Input: dimensioned drawing with shaded views. Units: mm. Origin: part minimum x, y, z. Coordinates: 2 decimals unless noted, no trailing zeros. Order: outer loops, then holes, each group sorted by start corner. A loop starts at its lowest first (then second) coordinate and runs counter-clockwise, first axis right, second up. Notation, with made-up numbers: (-33.75, 51.25) -> (-11.75, 51.25) arc R4 ccw to (-11.75, 56.25) -> close; hole circle Ø7 at (7, 16). An arc over 180 degrees is marked (long way). Answer in a Markdown table with one row per item. Add a question column.
1) Section query A-A on x = 50.8. Return the cut outline in (y, z).
2) Section query B-B on y = 19.05. Count the separate pieces of the cut face and the enclosed holes in it.
3) Ray query, line 1 (X direction, y = 19.05, z = 14.25); line 2 (X direction, y = 18, z = 15.5); line 3 (Z direction, x = 127, y = 3.5) (1 decimal). Return the intervals inside material, ascending. Write a range as from..to.
4) Contact query for a flat-ended pin moving along its axis: P1, Ø1, axis at x = 179.5, z = 11, coming from the -Y side. Output: stop coordinate, or through.
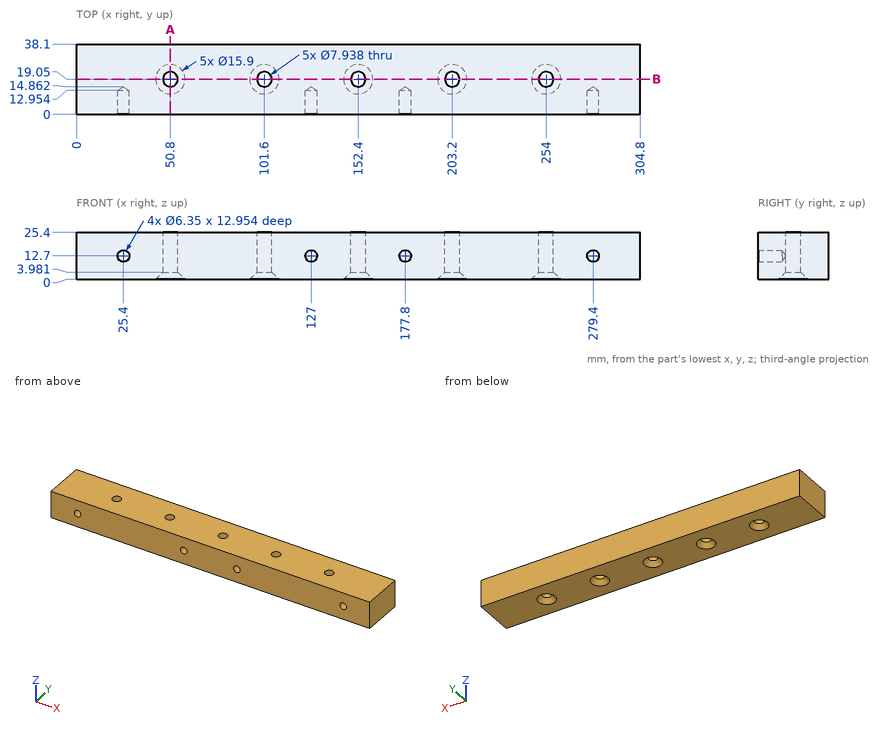
Result:
| question | item | result |
|---|---|---|
| 1 | outline | (0, 0) -> (11.1, 0) -> (15.08, 3.98) -> (15.08, 25.4) -> (0, 25.4) -> close; (23.02, 3.98) -> (27, 0) -> (38.1, 0) -> (38.1, 25.4) -> (23.02, 25.4) -> close |
| 2 | separate pieces | 6 |
| 2 | enclosed holes | 0 |
| 3 | line 1 | 0..46.83, 54.77..97.63, 105.57..148.43, 156.37..199.23, 207.17..250.03, 257.97..304.8 |
| 3 | line 2 | 0..46.97, 54.63..97.77, 105.43..148.57, 156.23..199.37, 207.03..250.17, 257.83..304.8 |
| 3 | line 3 | 0..9.5, 15.9..25.4 |
| 4 | P1 | y = 13.12 |
